The listing builds one solid part. Answer for the finished solid, in the listing's coordinates (mm). Face numbers are marked on the shaded views. A direction names the side the tool comes from. Coordinates: 2 decimals unless noted, no trailing zeros. Loops run counter-clockwise (first coordinate to the right, second up) from the corner with the lowest first, then second, coordinate; pieces in that order, holes last. Notation, with made-up numbers: (41, 0.5) -> (98, 0.5) arc R36 cw to (98, 35.5) -> close; hole circle Ø11 at (4, 32). An arc over 180 degrees is marked (long way). Answer in a Markdown table with one row per item.
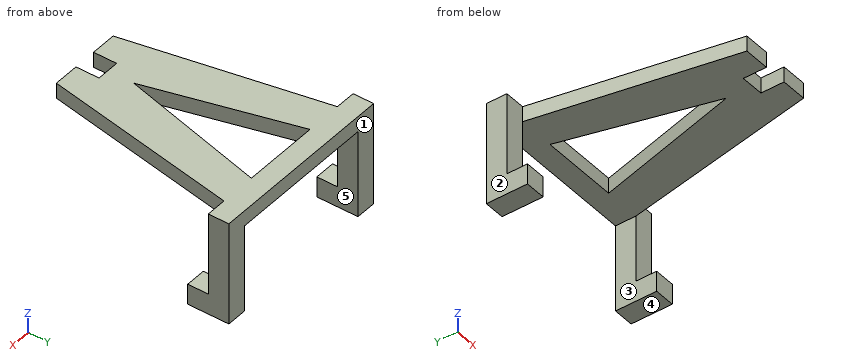
```python
from build123d import *

# Parameters (mm, degrees)
F1_DEPTH = 3
F3_START = 14.5
F2_W     = 4
F2_H     = 13
F3_DEPTH = 4
F6_DEPTH = 25


# Not quite as in the source:
# - a feature names something its author has since deleted; it is built from what else it names


with BuildPart() as f1:
    # F0 (on Top) → F1 (new body)
    with BuildSketch(Plane.XY):
        Polygon((-18.5, 17.05), (-14.5, 17.05), (14.5, 17.05), (18.5, 17.05), (18.5, 21.05), (-18.5, 21.05), align=None)
        Polygon((14.5, 17.05), (-14.5, 17.05), (-7.25, -21.05), (-2.25, -21.05), (-2.25, -16.55), (2.25, -16.55), (2.25, -21.05), (7.25, -21.05), align=None)
    extrude(amount=F1_DEPTH)

    # F2 (on Right) → F3 (join)
    with BuildSketch(Plane.YZ.offset(F3_START)):
        with Locations((19.05, -6.5)):
            Rectangle(F2_W, F2_H)
        Polygon((21.05, -17), (21.05, -13), (17.05, -13), (13.05, -13), (13.05, -17), align=None)
    extrude(amount=F3_DEPTH)

    # F4: F1 across plane


with BuildPart() as f1_1:
    add(f1.part)
    add(f1.part.mirror(Plane.YZ))

    # F5 (on Top) → F6 (cut)
    with BuildSketch(Plane.XY):
        Polygon((7.5, 17.05), (-7.5, 17.05), (0, -11.55), align=None)
    extrude(amount=F6_DEPTH, mode=Mode.SUBTRACT)


solid = f1_1.part
```
Item 1: A cutting plane is placed at A-A, the plane z = -3. Determine the outline of the cut face in (x, y).
Findings below:
| item | result |
|---|---|
| outline | (-18.5, 17.05) -> (-14.5, 17.05) -> (-14.5, 21.05) -> (-18.5, 21.05) -> close; (14.5, 17.05) -> (18.5, 17.05) -> (18.5, 21.05) -> (14.5, 21.05) -> close |
Item 2: A tool of negligible diameter and unlimited length cuts with its end or side. For the marked faces 4 and 5, from which of +Z, -Z, +X, -X, +Y, -Y can it reach the whole face along a straight path? Write none if from no direction.
Findings below:
| item | result |
|---|---|
| face 4 | -Z, +X, -X, +Y, -Y |
| face 5 | -Z, +Y, -Y |
Item 3: A cutting plane is placed at D-D, the plane x = 10.5. Determine the outline of the cut face in (y, z).
Findings below:
| item | result |
|---|---|
| outline | (-3.97, 0) -> (21.05, 0) -> (21.05, 3) -> (-3.97, 3) -> close |
Item 4: Flat-ended cylindrical pins translate along their axes: pin 1 Ø0.9 at (y, z) = (-19, 2) entering from -X; pin 2 Ø4.5 at (x, z) = (-17, -14) entering from -Y; pin 3 Ø1.2 at (x, z) = (16.5, -3) entering from -Y. Find the tip coordinate at first contact, or state that the pin passes through.
Findings below:
| item | result |
|---|---|
| pin 1 | stops at x = -7.73 |
| pin 2 | stops at y = 13.05 |
| pin 3 | stops at y = 17.05 |
Item 5: Find the intervals of material crossed by probe 1 along X at (y, z) = (18, -13.25); probe 2 along Z at (x, y) = (11, 17.5); probe 3 along X at (y, z) = (-2, 2.25) (3 decimals), in increasing order.
Findings below:
| item | result |
|---|---|
| probe 1 | x = -18.5 to -14.5, 14.5 to 18.5 |
| probe 2 | z = 0 to 3 |
| probe 3 | x = -10.875 to -2.504, 2.504 to 10.875 |
Item 6: Determine the mould class of the marked faces 1, 2 and 3 for opening direction X: +X half, -X half, draft (parallel to the pull), parting line (faces both ways), or undercut.
Findings below:
| item | result |
|---|---|
| face 1 | draft |
| face 2 | -X half |
| face 3 | undercut |
Item 7: A cutting plane is placed at B-B, the plane x = 6. Determine the outline of the cut face in (y, z).
Findings below:
| item | result |
|---|---|
| outline | (-21.05, 0) -> (11.33, 0) -> (11.33, 3) -> (-21.05, 3) -> close; (17.05, 0) -> (21.05, 0) -> (21.05, 3) -> (17.05, 3) -> close |
Item 8: A cutting plane is placed at C-C, the plane y = 18. Determine the outline of the cut face in (x, z).
Findings below:
| item | result |
|---|---|
| outline | (-18.5, -17) -> (-14.5, -17) -> (-14.5, 0) -> (14.5, 0) -> (14.5, -17) -> (18.5, -17) -> (18.5, 3) -> (-18.5, 3) -> close |
